Here's how the part is built. I have some questions about the finished solid (model axes, mm). A direction names the side the tool comes from. Give positions to 0.01 mm unless a question says otherwise; leave off trailing zeros. Write each loop counter-clockwise with the first axis right and the second up, starting at its lowest first coordinate (ties: lowest second). Pieces come first, ordered by that corner, then holes. Notation, with made-up numbers: M 21,54 L 26,54 A15 cw 26,73 Z; hole C -3.5,27 d2. An arc over 180 degrees is marked long. Answer as CSV lines item,"result". Start each with the question number.
Q1. If I drill on line 1 along Y through (x, z) = (36.5, 52); line 2 along X through (y, z) = (7, 35); line 3 along Z through (x, y) = (22, -15), over which ranges is the centre line in solid material (lowest first)?
Q2. Suppose I cut it at A-A (x = 26). Write out the boundary of the cut face in (y, z).
Q3. Suppose I cut it at C-C (z = -19). Write out the boundary of the cut face in (x, y).
Q4. Suppose I cut it at B-B (y = -15). Write out the boundary of the cut face in (x, z), then the cut area to 3 significant figures.
Q5. For pin 1 (10 mm diameter, centred on x = -3, y = -8, fed in from -Z); pin 2 (4 mm diameter, centred on x = 30, z = 15.5, fed in from +Y); pin 3 (15 mm diameter, centred on y = 12.5, z = -46, fed in from -X), each with a flat end and sliding along its axis, tell me the tip position at first contact or that it passes through.
Q6. On a 3-axis mill with a long thin cutter (end or side, diameter ignored), from which of +Z, -Z, +X, -X, +Y, -Y can I reach the whole of each face in a straight line? I mean faces 1 (the flat face through (-1, 5, 127.5)), 2 (the flat face through (1, 30, -34)), 3 (the flat face through (1, 0, -34)), 4 (the flat face through (-1, -22, 92)), 5 (the flat face through (-57.5, 15, -36)). Say none if no direction works.
Autodesk Inventor part; units mm, degrees
ref_plane "YZ Plane" through (0, 0, 0) normal (1, 0, 0) x (0, 1, 0)
ref_plane "XZ Plane" through (0, 0, 0) normal (0, 1, 0) x (-1, 0, 0)
ref_plane "XY Plane" through (0, 0, 0) normal (0, 0, 1) x (1, 0, 0)
sketch "Sketch1" plane through (0, 0, 0) normal (0, 1, 0) x (-1, 0, 0)
  line L0 (-57.5, -127.5) -> (57.5, -127.5)
  line L1 (57.5, -127.5) -> (57.5, 127.5)
  line L2 (57.5, 127.5) -> (-57.5, 127.5)
  line L3 (-57.5, 127.5) -> (-57.5, -127.5)
  line L4 (-57.5, -127.5) -> (57.5, 127.5) construction
  line L5 (57.5, -127.5) -> (-57.5, 127.5) construction
  point P0 (0, 0)
  dimension "d0" = 115
  dimension "d1" = 255
extrude "Extrusion1" add sketch "Sketch1" along normal blind 30
sketch "Sketch2" plane through (0, 30, 0) normal (0, 1, 0) x (1, 0, 0)
  line L0 (-57.5, -127.5) -> (57.5, -127.5)
  line L1 (58.5, -57.5) -> (-58.5, -57.5)
  line L2 (-58.5, -57.5) -> (-58.5, -127.5)
  line L3 (-58.5, -127.5) -> (58.5, -127.5)
  line L4 (58.5, -127.5) -> (58.5, -57.5)
  line L5 (58.5, -57.5) -> (-58.5, -127.5) construction
  line L6 (-58.5, -57.5) -> (58.5, -127.5) construction
  line L7 (57.5, -57.5) -> (57.5, -127.5)
  point P0 (0, 0)
  point P1 (0, -92.5)
  dimension "d4" = 35
  dimension "d5" = 117
extrude "Extrusion2" add sketch "Sketch2" along normal blind 2 contours L3 L2 L1 L7 L0
extrude "Extrusion3" add sketch "Sketch2" against normal blind 52 contours L3 L2 L1 L7 L0
properties part number "PSU"
Resolved:
1,line 1,"0 to 30"
1,line 2,"-57.5 to 57.5"
1,line 3,"57.5 to 127.5"
2,outline,"M -22,57.5 L 0,57.5 L 0,-127.5 L 30,-127.5 L 30,57.5 L 32,57.5 L 32,127.5 L -22,127.5 Z"
3,outline,"M -57.5,0 L 57.5,0 L 57.5,30 L -57.5,30 Z"
4,outline,"M -58.5,57.5 L 57.5,57.5 L 57.5,127.5 L -58.5,127.5 Z"
4,area,"8,120 mm^2"
5,pin 1,"z = 57.5"
5,pin 2,"y = 30"
5,pin 3,"x = -57.5"
6,face 1,"+Z, +X, -X, +Y, -Y"
6,face 2,"-Z, +X, -X, +Y"
6,face 3,"-Z, +X, -X, -Y"
6,face 4,"+Z, -Z, +X, -X, -Y"
6,face 5,"-Z, -X, +Y, -Y"
